The drawing under review shows one solid part. Ordinate dimensions are in mm from its lowest x, y, z. A direction names the side the tool comes from. Round coordinates to 2 decimals unless told otherwise and drop trailing zeros. Write each loop counter-clockwise with the first axis right and the second up, starting at its lowest first coordinate (ties: lowest second). Pieces come first, ordered by that corner, then holes.
Item 1: Add section A-A (x = 44). Give the boundary of the cut face in (y, z).
Item 2: To check wall thickness, follow L1, parallel to Y at x = 147.5, z = 50.65; L2, parallel to X at y = 52.7, z = 2.5; L3, parallel to Z at x = 147.5, y = 53.55. State the ranges of each line that lie inside material, in increasing order.
Item 3: Machinability: for the marked faces 1 and 2, which of the approach directions +Z, -Z, +X, -X, +Y, -Y give a long, thin tool a straight path to every point of the face, cutting with its end or side? Answer none if there is none.
Item 4: Clearance check with flat-ended pins moving along their axes: pin 1 Ø3 at (x, y) = (2.5, 49.5) entering from -Z; pin 2 Ø10 at (x, z) = (111.5, 30) entering from -Y; pin 3 Ø1.6 at (x, y) = (111.5, 53) entering from -Z. State where each tip first meets the part, or that it passes through.
Item 5: Add section B-B (y = 42.5). Give the boundary of the cut face in (x, z).
Item 6: Add section C-C (z = 22). Give the boundary of the cut face in (x, y), plus the area to 3 significant figures.
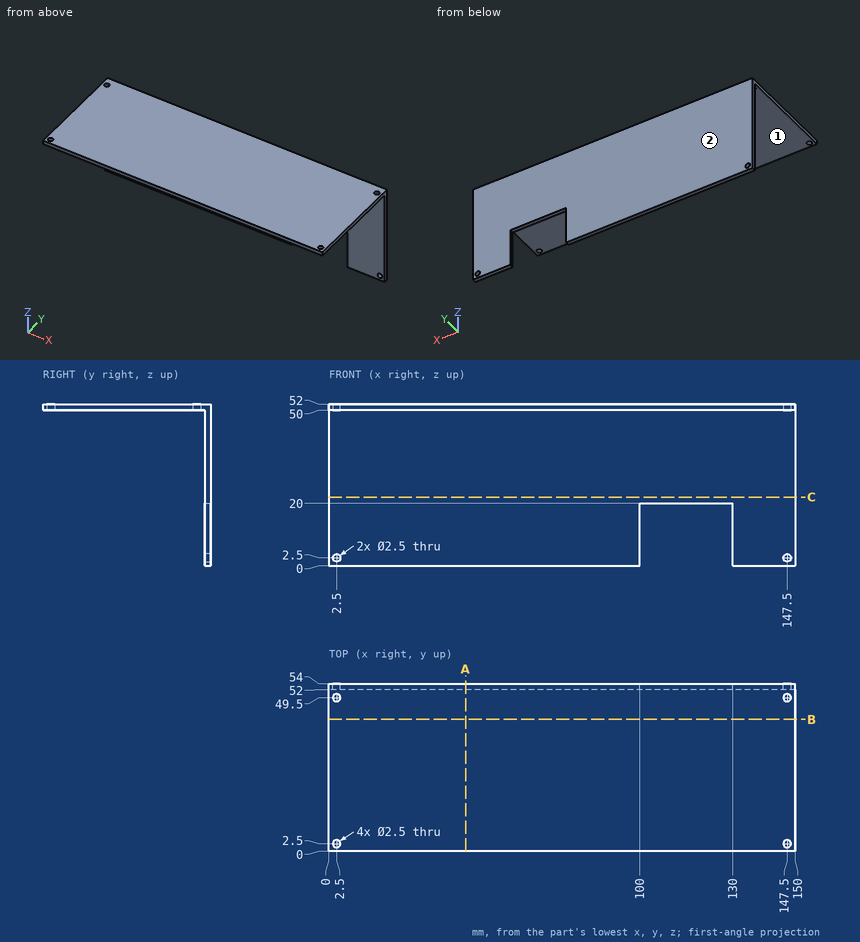
Numbers:
1. outline: (0, 50) - (52, 50) - (52, 0) - (54, 0) - (54, 52) - (0, 52) - close
2. L1: y = 0 to 1.25, 3.75 to 48.25, 50.75 to 54
2. L2: x = 0 to 1.25, 3.75 to 100, 130 to 146.25, 148.75 to 150
2. L3: z = 0 to 1.25, 3.75 to 52
3. face 1: -Z, +X, -X, -Y
3. face 2: +Z, -Z, +X, -X, +Y
4. pin 1: stops at z = 50
4. pin 2: stops at y = 52
4. pin 3: stops at z = 20
5. outline: (0, 50) - (150, 50) - (150, 52) - (0, 52) - close
6. outline: (0, 52) - (150, 52) - (150, 54) - (0, 54) - close
6. area: 300 mm2
